Design review of the part built by this model. Coordinates are the model's own, in mm. Face numbers are marked on the shaded views. A direction names the side the tool comes from. Round coordinates to 2 decimals unless told otherwise and drop trailing zeros. Order: outer loops, then holes, each group sorted by start corner. A loop starts at its lowest first (then second) coordinate and runs counter-clockwise, first axis right, second up. Notation, with made-up numbers: M 24,-17.5 L 69,-17.5 A10 ccw 69,0.5 Z; hole C 81,44 d10. An arc over 180 degrees is marked long. Use a Markdown table: item, result. Add a question column.
(1) Take a section at B-B (y = -4.25). Write out the cut boundary in (x, z).
(2) Take a section at A-A (z = 2.75). Write out the cut boundary in (x, y).
(3) The part is to be moulded in two halves that separate along X. For the marked faces 6, 7 and 8, say which applies: released by +X, released by -X, zero draft, split by the parting line, or undercut.
(4) To check wall thickness, follow probe 1 along X at (y, z) = (-6.5, 9.25); probe 2 along Y at (x, z) = (5, 4.75); probe 3 along Z at (x, y) = (0.5, 2.5). State the ranges of each line that lie inside material, in increasing order. Write a range as from..to.
(5) Machinability: for the marked faces 1, 2, 3, 4 and 5, which of the approach directions +Z, -Z, +X, -X, +Y, -Y give a long, thin tool a straight path to every point of the face, cutting with its end or side? Answer none if there is none.
(6) Take a section at D-D (z = 5.5). Write out the cut boundary in (x, y).
(7) For pin 1 (1.8 mm diameter, centred on x = 4.5, z = 3, fed in from -Y); pin 2 (6 mm diameter, centred on y = -1, z = 11, fed in from +X); pin 3 (4.5 mm diameter, centred on x = 0.5, y = 4, fed in from +Z), all flat-tipped, find the tip position at first contact; note any pin that passes through.
(8) Take a section at C-C (x = 1.75). Write out the cut boundary in (y, z).
```python
from build123d import *

# Parameters (mm, degrees)
F1_DEPTH    = 19.304
F0_W        = 4.2467024177
F0_H        = 13.0065511912
F2_DEPTH    = 6.096
F3_T1_DEPTH = 6.096
F3_T3_DEPTH = 6.096
F3_T5_DEPTH = 19.1620992743
F3_T7_DEPTH = 19.1620992743
F3_T9_DEPTH = 28.0302021899


# Not quite as in the source:
# - a fillet or chamfer that OpenCascade refuses, or shapes differently, is made with other operations: its cross-section is extruded or revolved along the edge and cut away or added


with BuildPart() as f1:
    # F0 (on Top) → F1 (new body)
    with BuildSketch(Plane.XY):
        Polygon((-6.1091380194, 8.0798277631), (-6.1091380194, 0), (-6.1091380194, -8.0798277631), (-1.9706897438, -8.0798277631), (-1.9706897438, -6.5032755956), (-1.9706897438, 6.5032755956), (-1.9706897438, 8.0798277631), align=None)
    extrude(amount=F1_DEPTH)

    # F0 (on Top) → F2 (join)
    with BuildSketch(Plane.XY):
        with Locations((0.1526614651, 0)):
            Rectangle(F0_W, F0_H)
        with Locations((4.3993638828, 0)):
            Rectangle(F0_W, F0_H)
    extrude(amount=F2_DEPTH)

    # F3: fillet of radius 3.0047301997 on 5 edges, made by hand

    # F3_s2 → F3_t1 (join)
    with BuildSketch(Plane.XY):
        with BuildLine():
            ThreePointArc((-1.9706897438, -8.0798277631), (-0.8660843797, -6.9273379324), (0.6729273014, -6.5032755956))
            Line((0.6729273014, -6.5032755956), (-1.9706897438, -6.5032755956))
            Line((-1.9706897438, -6.5032755956), (-1.9706897438, -8.0798277631))
        make_face()
    extrude(amount=F3_T1_DEPTH)

    # F3_s4 → F3_t3 (join)
    with BuildSketch(Plane.XY):
        with BuildLine():
            ThreePointArc((-1.9706897438, 8.0798277631), (-0.8660843797, 6.9273379324), (0.6729273014, 6.5032755956))
            Line((0.6729273014, 6.5032755956), (-1.9706897438, 6.5032755956))
            Line((-1.9706897438, 6.5032755956), (-1.9706897438, 8.0798277631))
        make_face()
    extrude(amount=F3_T3_DEPTH)

    # F3_s6 → F3_t5 (cut)
    with BuildSketch(Plane.YZ.offset(-13.6209635187)):
        with BuildLine():
            ThreePointArc((5.0750975634, 19.304), (7.1997626633, 18.4239349001), (8.0798277631, 16.2992698003))
            Line((8.0798277631, 16.2992698003), (8.0798277631, 19.304))
            Line((8.0798277631, 19.304), (5.0750975634, 19.304))
        make_face()
    extrude(amount=F3_T5_DEPTH, mode=Mode.SUBTRACT)

    # F3_s8 → F3_t7 (cut)
    with BuildSketch(Plane.YZ.offset(-13.6209635187)):
        with BuildLine():
            ThreePointArc((-8.0798277631, 16.2992698003), (-7.1997626633, 18.4239349001), (-5.0750975634, 19.304))
            Line((-5.0750975634, 19.304), (-8.0798277631, 19.304))
            Line((-8.0798277631, 19.304), (-8.0798277631, 16.2992698003))
        make_face()
    extrude(amount=F3_T7_DEPTH, mode=Mode.SUBTRACT)

    # F3_s10 → F3_t9 (cut)
    with BuildSketch(Plane.XZ.offset(-14.0151010949)):
        with BuildLine():
            ThreePointArc((6.5227150917, 3.0912698003), (5.6426499918, 5.2159349001), (3.517984892, 6.096))
            Line((3.517984892, 6.096), (6.5227150917, 6.096))
            Line((6.5227150917, 6.096), (6.5227150917, 3.0912698003))
        make_face()
    extrude(amount=F3_T9_DEPTH, mode=Mode.SUBTRACT)


solid = f1.part
```
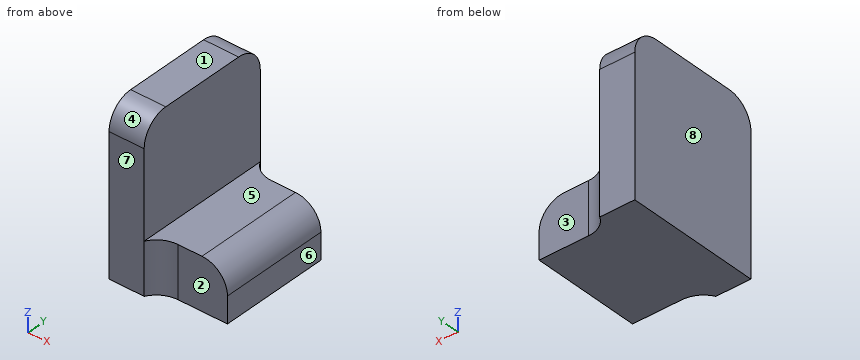
Verdict:
| question | item | result |
|---|---|---|
| 1 | outline | M -6.11,0 L 6.52,0 L 6.52,3.09 A3 ccw 3.52,6.1 L -1.97,6.1 L -1.97,19.3 L -6.11,19.3 Z |
| 2 | outline | M -6.11,-8.08 L -1.97,-8.08 A3 cw 0.67,-6.5 L 6.52,-6.5 L 6.52,6.5 L 0.67,6.5 A3 cw -1.97,8.08 L -6.11,8.08 Z |
| 3 | face 6 | released by +X |
| 3 | face 7 | zero draft |
| 3 | face 8 | released by -X |
| 4 | probe 1 | x = -6.11..-1.97 |
| 4 | probe 2 | y = -6.5..6.5 |
| 4 | probe 3 | z = 0..6.1 |
| 5 | face 1 | +Z, +X, -X, +Y, -Y |
| 5 | face 2 | +Z, -Z, +X, -Y |
| 5 | face 3 | +Z, -Z, +X, +Y |
| 5 | face 4 | +Z, +X, -X, -Y |
| 5 | face 5 | +Z, +X, +Y, -Y |
| 6 | outline | M -6.11,-8.08 L -1.97,-8.08 A3 cw 0.67,-6.5 L 5.31,-6.5 L 5.31,6.5 L 0.67,6.5 A3 cw -1.97,8.08 L -6.11,8.08 Z |
| 7 | pin 1 | stops at y = -6.5 |
| 7 | pin 2 | stops at x = -1.97 |
| 7 | pin 3 | stops at z = 6.1 |
| 8 | outline | M -6.5,0 L 6.5,0 L 6.5,6.1 L -6.5,6.1 Z |
